Work out the finished part from the listing and answer in its coordinate system (mm). A direction names the side the tool comes from. Give positions to 0.01 mm unless a question says otherwise; leave off trailing zeros. Loops run counter-clockwise (first coordinate to the right, second up) from the corner with the lowest first, then second, coordinate; pieces in that order, holes last. Notation, with made-up numbers: (-27, 39.5) - (31, 39.5) arc R23 cw to (31, 66.5) - close; hole circle Ø9 at (66, -11.75). An arc over 180 degrees is marked (long way). One line per question, with ' | ' between items. Start each with the question number.
1. Each of these flat-tipped pins is pushed along its axis until it touches: pin 1 (8 mm diameter, centred on x = 7, y = 36.5, fed in from +Z); pin 2 (1.1 mm diameter, centred on x = 7.5, z = 11.5, fed in from +Y); pin 3 (6 mm diameter, centred on x = 7, z = -6, fed in from +Y); pin 4 (1.8 mm diameter, centred on x = 0, y = 39.751, fed in from -Z). Where does it stop, or does it pass through?
2. Section D-D (y = -8.5) is taken. Determine the outline of the cut face in (x, z), plus the area to 3 significant figures.
3. Section A-A (x = 0) is taken. Give the number of separate pieces and of enclosed holes in the cut face, plus the area to 3 significant figures.
4. Section C-C (x = -9.25) is taken. Determine the outline of the cut face in (y, z), plus the area to 3 significant figures.
5. Section B-B (z = 0) is taken. Determine the outline of the cut face in (x, y), plus the area to 3 significant figures.
6. Which of the six approach directions +Z, -Z, +X, -X, +Y, -Y give full straight-line access (tool end or side, diameter ignored) to faces 1 (the face through (-8.4, 25.4, -10.287)), 2 (the face through (5.702, 25.4, 11.4)), 3 (the face through (-8, 26.01, -11))?
7. For a pull along Z with two mould halves and no side action, classify faces 4 (the face through (6.117, 25.543, -1.926)), 5 (the face through (0, 14, 12.548)), 6 (the face through (0, -12.497, 0)), 7 (the face through (-1, 38, 1.321)) as released by +Z, released by -Z, zero draft, split by the parting line, or undercut.
8. Find the intervals of material crossed by line 1 (Z direction, x = 0, y = 25.35); line 2 (Y direction, x = 0, z = 2.85), in increasing order.
from build123d import *

# Parameters (mm, degrees)
SKETCH1_W                      = 22.225
SKETCH1_H                      = 25.0952
BOSS_EXTRUDE1_DEPTH            = 24.8666
SKETCH2_R                      = 3.0226
BOSS_EXTRUDE2_DEPTH            = 12.496800002
SKETCH3_R                      = 3.7592
BOSS_EXTRUDE3_DEPTH            = 18.288000094
SKETCH4_R                      = 7.6835
SKETCH4_R_2                    = 6.4135
BOSS_EXTRUDE4_DEPTH            = 1.3716
SKETCH5_W                      = 5.4102
SKETCH5_H                      = 2.2606
BOSS_EXTRUDE5_DEPTH            = 1.143
FILLET1_R                      = 2.54
CUT_EXTRUDE1_REACH             = 13.113
SKETCH6_W                      = 2.6416
SKETCH6_H                      = 7.9248
CUT_EXTRUDE1_DIRECTION_2_REACH = 13.112
CUT_EXTRUDE2_REACH             = 14.548
SKETCH7_R                      = 1.4986
CUT_EXTRUDE2_DIRECTION_2_REACH = 14.548


with BuildPart() as part:
    # Sketch1 → Boss-Extrude1 (new body)
    with BuildSketch(Plane(origin=(0, 0, 0), x_dir=(1, 0, 0), z_dir=(0, 1, 0))):
        Rectangle(SKETCH1_W, SKETCH1_H)
    extrude(amount=BOSS_EXTRUDE1_DEPTH)

    # Sketch2 → Boss-Extrude2 (add)
    with BuildSketch(Plane.XZ):
        Circle(SKETCH2_R)
    extrude(amount=BOSS_EXTRUDE2_DEPTH)

    # Sketch3 → Boss-Extrude3 (add)
    with BuildSketch(Plane(origin=(0, 24.8666, 0), x_dir=(1, 0, 0), z_dir=(0, 1, 0))):
        Circle(SKETCH3_R)
    extrude(amount=BOSS_EXTRUDE3_DEPTH)

    # Sketch4 → Boss-Extrude4 (add)
    with BuildSketch(Plane(origin=(0, 24.8666, 0), x_dir=(1, 0, 0), z_dir=(0, 1, 0))):
        Circle(SKETCH4_R)
        Circle(SKETCH4_R_2, mode=Mode.SUBTRACT)
    extrude(amount=BOSS_EXTRUDE4_DEPTH)

    # Sketch5 → Boss-Extrude5 (add)
    with BuildSketch(Plane(origin=(0, 24.8666, 0), x_dir=(1, 0, 0), z_dir=(0, 1, 0))):
        with Locations((-8.4074, -11.4173)):
            Rectangle(SKETCH5_W, SKETCH5_H)
        with Locations((8.4074, -11.4173)):
            Rectangle(SKETCH5_W, SKETCH5_H)
        with Locations((8.4074, 11.4173)):
            Rectangle(SKETCH5_W, SKETCH5_H)
        with Locations((-8.4074, 11.4173)):
            Rectangle(SKETCH5_W, SKETCH5_H)
    extrude(amount=BOSS_EXTRUDE5_DEPTH)

    # Fillet1
    fillet1_edges = [part.edges().sort_by_distance(p)[0] for p in [
        (0, 0, 12.5476),
        (0, 0, -12.5476),
    ]]
    fillet(fillet1_edges, radius=FILLET1_R)

    # Sketch6 → Cut-Extrude1 (cut, up to next)
    with BuildSketch(Plane(origin=(0, 0, 0), x_dir=(0, 0, -1), z_dir=(1, 0, 0)), mode=Mode.PRIVATE) as cut_extrude1_sk1:
        with Locations((0, 39.192200094)):
            Rectangle(SKETCH6_W, SKETCH6_H)
    cut_extrude1_tool1 = extrude(cut_extrude1_sk1.sketch, amount=-CUT_EXTRUDE1_REACH, mode=Mode.PRIVATE) & part.part
    add(cut_extrude1_tool1.solids().sort_by_distance((0, 39.1922, 0))[0], mode=Mode.SUBTRACT)

    # Sketch6 → Cut-Extrude1 direction 2 (cut, up to next)
    with BuildSketch(Plane(origin=(0, 0, 0), x_dir=(0, 0, -1), z_dir=(1, 0, 0)), mode=Mode.PRIVATE) as cut_extrude1_direction_2_sk1:
        with Locations((0, 39.192200094)):
            Rectangle(SKETCH6_W, SKETCH6_H)
    cut_extrude1_direction_2_tool1 = extrude(cut_extrude1_direction_2_sk1.sketch, amount=CUT_EXTRUDE1_DIRECTION_2_REACH, mode=Mode.PRIVATE) & part.part
    add(cut_extrude1_direction_2_tool1.solids().sort_by_distance((0, 39.1922, 0))[0], mode=Mode.SUBTRACT)

    # Sketch7 → Cut-Extrude2 (cut, up to next)
    with BuildSketch(Plane.XY, mode=Mode.PRIVATE) as cut_extrude2_sk1:
        with Locations((0, 39.751000094)):
            Circle(SKETCH7_R)
    cut_extrude2_tool1 = extrude(cut_extrude2_sk1.sketch, amount=-CUT_EXTRUDE2_REACH, mode=Mode.PRIVATE) & part.part
    add(cut_extrude2_tool1.solids().sort_by_distance((0, 39.751, 0))[0], mode=Mode.SUBTRACT)

    # Sketch7 → Cut-Extrude2 direction 2 (cut, up to next)
    with BuildSketch(Plane.XY, mode=Mode.PRIVATE) as cut_extrude2_direction_2_sk1:
        with Locations((0, 39.751000094)):
            Circle(SKETCH7_R)
    cut_extrude2_direction_2_tool1 = extrude(cut_extrude2_direction_2_sk1.sketch, amount=CUT_EXTRUDE2_DIRECTION_2_REACH, mode=Mode.PRIVATE) & part.part
    add(cut_extrude2_direction_2_tool1.solids().sort_by_distance((0, 39.751, 0))[0], mode=Mode.SUBTRACT)


solid = part.part
Conclusion:
1) pin 1: z = 2.27 | pin 2: y = 26.01 | pin 3: y = 26.24 | pin 4: through
2) outline: circle Ø6.05 at (0, 0) | area: 28.7 mm²
3) separate pieces: 3 | enclosed holes: 0 | area: 802 mm²
4) outline: (0, -10.01) arc R2.54 ccw to (2.54, -12.55) - (26.01, -12.55) - (26.01, -10.29) - (24.87, -10.29) - (24.87, 10.29) - (26.01, 10.29) - (26.01, 12.55) - (2.54, 12.55) arc R2.54 ccw to (0, 10.01) - close | area: 626 mm²
5) outline: (-11.11, 0) - (-3.02, 0) - (-3.02, -12.5) - (3.02, -12.5) - (3.02, 0) - (11.11, 0) - (11.11, 24.87) - (7.68, 24.87) - (7.68, 26.24) - (6.41, 26.24) - (6.41, 24.87) - (3.76, 24.87) - (3.76, 35.23) - (-3.76, 35.23) - (-3.76, 24.87) - (-6.41, 24.87) - (-6.41, 26.24) - (-7.68, 26.24) - (-7.68, 24.87) - (-11.11, 24.87) - close | area: 710 mm²
6) face 1: +X, -X, +Y | face 2: +Z, +Y | face 3: -Z, +X, -X, +Y
7) face 4: undercut | face 5: released by +Z | face 6: zero draft | face 7: undercut
8) line 1: -7.68 to -6.41, -3.76 to 3.76, 6.41 to 7.68 | line 2: -12.5 to 38.25, 41.25 to 43.15
